```python
from build123d import *

# Parameters (mm, degrees)
SKETCH_1_W      = 35
SKETCH_1_H      = 35
SKETCH_1_R      = 1.5
SKETCH_1_R_2    = 6
SKETCH_1_R_3    = 1.4
EXTRUDE_1_DEPTH = 5
FILLET_1_R      = 5


with BuildPart() as part:
    # 草图1 → 凸台-拉伸1 (new body)
    with BuildSketch(Plane.XY):
        Rectangle(SKETCH_1_W, SKETCH_1_H)
        with Locations((0, 12.5)):
            Circle(SKETCH_1_R, mode=Mode.SUBTRACT)
        with Locations((12.5, 0)):
            Circle(SKETCH_1_R, mode=Mode.SUBTRACT)
        with Locations((0, -12.5)):
            Circle(SKETCH_1_R, mode=Mode.SUBTRACT)
        with Locations((-12.5, 0)):
            Circle(SKETCH_1_R, mode=Mode.SUBTRACT)
        Circle(SKETCH_1_R_2, mode=Mode.SUBTRACT)
        with Locations((-7.5, 7.5)):
            Circle(SKETCH_1_R_3, mode=Mode.SUBTRACT)
        with Locations((7.5, 7.5)):
            Circle(SKETCH_1_R_3, mode=Mode.SUBTRACT)
        with Locations((7.5, -7.5)):
            Circle(SKETCH_1_R_3, mode=Mode.SUBTRACT)
        with Locations((-7.5, -7.5)):
            Circle(SKETCH_1_R_3, mode=Mode.SUBTRACT)
    extrude(amount=EXTRUDE_1_DEPTH)

    # 圆角1
    fillet_1_edges = [part.edges().sort_by_distance(p)[0] for p in [
        (17.5, -17.5, 2.5),
        (-17.5, -17.5, 2.5),
        (-17.5, 17.5, 2.5),
        (17.5, 17.5, 2.5),
    ]]
    fillet(fillet_1_edges, radius=FILLET_1_R)


solid = part.part
```
CAD build for the part. Positions are in the model's coordinates, mm. Give positions to 0.01 mm unless a question says otherwise; leave off trailing zeros. Write each loop counter-clockwise with the first axis right and the second up, starting at its lowest first coordinate (ties: lowest second). Pieces come first, ordered by that corner, then holes. Notation, with made-up numbers: M 81,-18.5 L 104,-18.5 A23 cw 104,-9.5 Z; hole C 63,-37.75 d5. An arc over 180 degrees is marked long. Return JSON: item names as keys, results as strings. Group by question number.
(1) Mould opens along Y. For faces 1 (the face through (-16.07, 16, 2.54)), 2 (the face through (-17.5, 0, 2)), 3 (the face through (0, 11, 2)) say: pulls with the +Y half, pulls with the -Y half, needs draft (parallel to the pull), parting line crosses it, or undercut.
(2) Band-saw the part on B-B (y = 7.5). Give the cut face in (x, z).
(3) Flat gauge pins, fed straight in: pin 1 Ø3.5 at (x, y) = (0, -12.5) entering from +Z; pin 2 Ø2.5 at (x, y) = (-7.5, -7.5) entering from -Z. Where does each tip first touch, or does it go through?
(4) Band-saw the part on C-C (z = 4.45). State how many separate pieces and enclosed holes the cut face has, and give its area (3 significant figures).
(5) Band-saw the part on A-A (x = 0). Give the cut face in (y, z).
(6) Drill centre lines: L1, parallel to Y at x = 0, z = 3.8; L2, parallel to Y at x = 8, z = 4.45; L3, parallel to X at y = 1, z = 4.05. Where is each one in solid material? Low to high. Write a range as [from, to].
Entries:
{
 "1": {"face 1": "pulls with the +Y half", "face 2": "needs draft", "face 3": "undercut"},
 "2": {"outline": "M -17.5,0 L -8.9,0 L -8.9,5 L -17.5,5 Z; M -6.1,0 L 6.1,0 L 6.1,5 L -6.1,5 Z; M 8.9,0 L 17.5,0 L 17.5,5 L 8.9,5 Z"},
 "3": {"pin 1": "stops at z = 5", "pin 2": "passes through"},
 "4": {"separate pieces": "1", "enclosed holes": "9", "area": "1,040 mm^2"},
 "5": {"outline": "M -17.5,0 L -14,0 L -14,5 L -17.5,5 Z; M -11,0 L -6,0 L -6,5 L -11,5 Z; M 6,0 L 11,0 L 11,5 L 6,5 Z; M 14,0 L 17.5,0 L 17.5,5 L 14,5 Z"},
 "6": {"L1": "y = [-17.5, -14], [-11, -6], [6, 11], [14, 17.5]", "L2": "y = [-17.5, -8.81], [-6.19, 6.19], [8.81, 17.5]", "L3": "x = [-17.5, -13.62], [-11.38, -5.92], [5.92, 11.38], [13.62, 17.5]"}
}
